Part model, mm, in its own coordinate system. Give positions to 0.01 mm unless a question says otherwise; leave off trailing zeros. Write each loop counter-clockwise with the first axis right and the second up, starting at its lowest first coordinate (ties: lowest second). Pieces come first, ordered by that corner, then holes. Notation, with made-up numbers: M 23,27.5 L 44,27.5 A27 ccw 44,46.5 Z; hole C 13,2.25 d9. An arc over 180 degrees is marked long. Use a Markdown table: item, result. Add a question column.
from build123d import *

# Parameters (mm, degrees)
SKETCH1_R           = 3.048
SKETCH1_R_2         = 1.4605
BOSS_EXTRUDE1_DEPTH = 20.574
SKETCH2_R           = 3.571875
BOSS_EXTRUDE2_DEPTH = 0.9525


with BuildPart() as part:
    # Sketch1 → Boss-Extrude1 (new body)
    with BuildSketch(Plane.XY):
        Circle(SKETCH1_R)
        Circle(SKETCH1_R_2, mode=Mode.SUBTRACT)
    extrude(amount=BOSS_EXTRUDE1_DEPTH)

    # Sketch2 → Boss-Extrude2 (add)
    with BuildSketch(Plane.XY.offset(20.574)):
        with Locations(Location((0, 0, 0), (0, 0, 180))):
            Circle(SKETCH2_R)
    extrude(amount=BOSS_EXTRUDE2_DEPTH)


solid = part.part
1. Cut at D-D (y = 2.5). Write the cut outline in (x, z), then the cut area to 3 significant figures.
2. Cut at C-C (z = 13.5). Write the cut outline in (x, y).
3. Flat gauge pin, fed straight in: pin 1 (0.9 mm diameter, centred on x = 0.5, y = 0.5, fed in from -Z). Where does the tip first touch, or does it go through?
4. Cut at A-A (x = 0). Write the cut outline in (y, z).
5. Cut at B-B (y = -1.75). Write the cut outline in (x, z), then the cut area to 3 significant figures.
6. Mould opens along X. For faces 1 (the cylindrical face through (-0.317, -1.426, 10.143)), 2 (the flat face through (0, 0, 21.527)), 3 (the cylindrical face through (-0.4, 3.02, 10.14)), 4 (the flat face through (0, 0, 20.574)) say: released by +X, released by -X, zero draft, split by the parting line, or undercut.
7. Drill centre lines: probe 1 along Y at (x, z) = (0, 5); probe 2 along Z at (x, y) = (-1, -0.5); probe 3 along Y at (x, z) = (1, 17.5). Where is each one in solid material? Low to high. Write a range as [from, to].
A:
| question | item | result |
|---|---|---|
| 1 | outline | M -2.55,20.57 L -1.74,20.57 L -1.74,0 L 1.74,0 L 1.74,20.57 L 2.55,20.57 L 2.55,21.53 L -2.55,21.53 Z |
| 1 | area | 76.6 mm² |
| 2 | outline | C 0,0 d6.1; hole C 0,0 d2.92 |
| 3 | pin 1 | stops at z = 20.57 |
| 4 | outline | M -3.57,20.57 L -3.05,20.57 L -3.05,0 L -1.46,0 L -1.46,20.57 L 1.46,20.57 L 1.46,0 L 3.05,0 L 3.05,20.57 L 3.57,20.57 L 3.57,21.53 L -3.57,21.53 Z |
| 5 | outline | M -3.11,20.57 L -2.5,20.57 L -2.5,0 L 2.5,0 L 2.5,20.57 L 3.11,20.57 L 3.11,21.53 L -3.11,21.53 Z |
| 5 | area | 109 mm² |
| 6 | face 1 | undercut |
| 6 | face 2 | zero draft |
| 6 | face 3 | split by the parting line |
| 6 | face 4 | undercut |
| 7 | probe 1 | y = [-3.05, -1.46], [1.46, 3.05] |
| 7 | probe 2 | z = [20.57, 21.53] |
| 7 | probe 3 | y = [-2.88, -1.06], [1.06, 2.88] |
